from build123d import *

# Parameters (mm, degrees)
SKETCH1_W              = 25.4
SKETCH1_H              = 44.45
SKETCH1_R              = 2.413
BOSS_EXTRUDE1_DEPTH    = 3.175
SKETCH2_W              = 25.4
SKETCH2_H              = 3.175
BOSS_EXTRUDE2_DEPTH    = 44.45
SKETCH3_R              = 2.413
CUT_EXTRUDE1_DEPTH     = 44.45
FILLET1_R              = 2.54
CONVERT_SOLID1_START   = -12.7
CONVERT_SOLID1_DEPTH   = 25.4
CONVERT_SOLID1_2_DEPTH = 25.4


# Read off the part's stored shape, not the designer's step: Convert-Solid1
with BuildPart() as part:
    # Sketch1 → Boss-Extrude1 (new body)
    with BuildSketch(Plane.XY):
        Rectangle(SKETCH1_W, SKETCH1_H)
        with Locations((0, 8.255)):
            Circle(SKETCH1_R, mode=Mode.SUBTRACT)
        with Locations((0.348627451, -10.795)):
            Circle(SKETCH1_R, mode=Mode.SUBTRACT)
    extrude(amount=BOSS_EXTRUDE1_DEPTH)

    # Sketch2 → Boss-Extrude2 (add)
    with BuildSketch(Plane.XY.offset(3.175)):
        with Locations((0, 20.6375)):
            Rectangle(SKETCH2_W, SKETCH2_H)
    extrude(amount=BOSS_EXTRUDE2_DEPTH)

    # Sketch3 → Cut-Extrude1 (cut)
    with BuildSketch(Plane(origin=(0, 22.225, 0), x_dir=(1, 0, 0), z_dir=(0, 1, 0))):
        with Locations(Location((0, -12.7, 0), (0, 0, 270))):
            Circle(SKETCH3_R)
        with Locations(Location((0, -31.75, 0), (0, 0, 270))):
            Circle(SKETCH3_R)
    extrude(amount=-CUT_EXTRUDE1_DEPTH, mode=Mode.SUBTRACT)

    # Fillet1
    fillet1_edges = [part.edges().sort_by_distance(p)[0] for p in [
        (-12.7, 20.6375, 47.625),
        (12.7, 20.6375, 47.625),
        (12.7, -22.225, 1.5875),
        (-12.7, -22.225, 1.5875),
    ]]
    fillet(fillet1_edges, radius=FILLET1_R)

    # Convert-Solid1 outline → Convert-Solid1 (cut)
    with BuildSketch(Plane.YZ.offset(CONVERT_SOLID1_START)):
        with BuildLine():
            Line((22.225, 0), (22.225, 5.555000066))
            ThreePointArc((22.225, 5.555000066), (20.59797815, 1.62702185), (16.669999934, 0))
            Line((16.669999934, 0), (22.225, 0))
        make_face()
    extrude(amount=CONVERT_SOLID1_DEPTH, mode=Mode.SUBTRACT)

    # Convert-Solid1 2 outline → Convert-Solid1 2 (add)
    with BuildSketch(Plane.YZ.offset(CONVERT_SOLID1_START)):
        with BuildLine():
            Line((19.05, 3.175), (19.05, 5.555000066))
            ThreePointArc((19.05, 5.555000066), (18.35291412, 3.87208588), (16.669999934, 3.175))
            Line((16.669999934, 3.175), (19.05, 3.175))
        make_face()
    extrude(amount=CONVERT_SOLID1_2_DEPTH)


solid = part.part
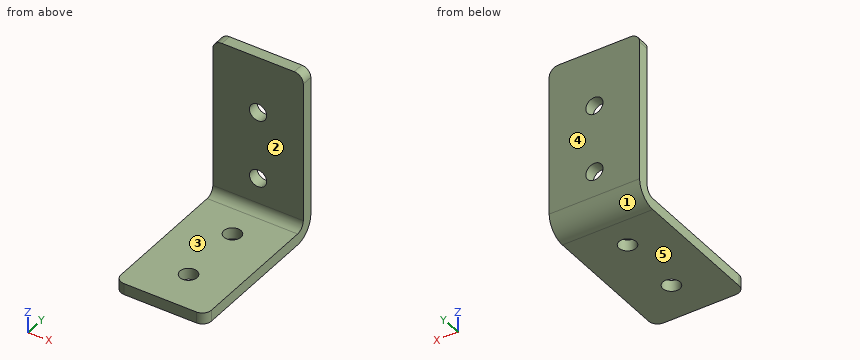
Verification items for the finished model (mm, model axes). Face numbers are marked on the shaded views. A direction names the side the tool comes from. Give positions to 0.01 mm unless a question says otherwise; leave off trailing zeros. Loops run counter-clockwise (first coordinate to the right, second up) from the corner with the lowest first, then second, coordinate; pieces in that order, holes last.
1) Draft check along Z on the marked faces 3, 4 and 5. Enter one of: pulls with the +Z half, pulls with the -Z half, needs draft (parallel to the pull), parting line crosses it, or undercut.
2) Set-up check for the marked faces 1 and 2: record each of +Z, -Z, +X, -X, +Y, -Y from which the full face is reachable in a straight line by a thin tool's end or side.
3) Sectioned sample at C-C, the plane x = 4.5. Enter the section's corners in (y, z) (3 decimals), then the cut area to 3 significant figures.
4) Sectioned sample at B-B, the plane x = 0. Enter the section's corners in (y, z) (3 decimals), then the cut area to 3 significant figures.
5) Sectioned sample at A-A, the plane z = 31.75. Enter the section's corners in (x, y) (3 decimals), then the cut area to 3 significant figures.
6) Thickness scan on line 1 along Y through (x, z) = (0, 2.4) (3 decimals); line 2 along Y through (x, z) = (0, 1.3) (3 decimals); line 3 along Z through (x, y) = (5, -3) (3 decimals). Record the ranges inside material, lowest first.
7) Depth check by flat-ended pin: pin 1 Ø7.5 at (x, z) = (0, 12.7) entering from -Y. Enter the tip coordinate at first touch or a pass-through.
8) Sectioned sample at D-D, the plane z = 14. Enter the section's corners in (x, y) (3 decimals), then the cut area to 3 significant figures.
Answers:
1. face 3: pulls with the +Z half
1. face 4: needs draft
1. face 5: pulls with the -Z half
2. face 1: -Z, +X, -X, +Y
2. face 2: +Z, +X, -X, -Y
3. outline: (-22.225, 0) - (16.67, 0) arc R5.555 ccw to (22.225, 5.555) - (22.225, 47.625) - (19.05, 47.625) - (19.05, 5.555) arc R2.38 cw to (16.67, 3.175) - (-22.225, 3.175) - close
3. area: 277 mm2
4. outline: (-22.225, 0) - (-13.183, 0) - (-13.183, 3.175) - (-22.225, 3.175) - close; (-8.407, 0) - (5.842, 0) - (5.842, 3.175) - (-8.407, 3.175) - close; (10.668, 0) - (16.67, 0) arc R5.555 ccw to (22.225, 5.555) - (22.225, 10.287) - (19.05, 10.287) - (19.05, 5.555) arc R2.38 cw to (16.67, 3.175) - (10.668, 3.175) - close; (19.05, 15.113) - (22.225, 15.113) - (22.225, 29.337) - (19.05, 29.337) - close; (19.05, 34.163) - (22.225, 34.163) - (22.225, 47.625) - (19.05, 47.625) - close
4. area: 216 mm2
5. outline: (-12.7, 19.05) - (-2.413, 19.05) - (-2.413, 22.225) - (-12.7, 22.225) - close; (2.413, 19.05) - (12.7, 19.05) - (12.7, 22.225) - (2.413, 22.225) - close
5. area: 65.3 mm2
6. line 1: y = -22.225 to -13.183, -8.407 to 5.842, 10.668 to 21.242
6. line 2: y = -22.225 to -13.183, -8.407 to 5.842, 10.668 to 20.241
6. line 3: z = 0 to 3.175
7. pin 1: stops at y = 19.05
8. outline: (-12.7, 19.05) - (-2.033, 19.05) - (-2.033, 22.225) - (-12.7, 22.225) - close; (2.033, 19.05) - (12.7, 19.05) - (12.7, 22.225) - (2.033, 22.225) - close
8. area: 67.7 mm2
